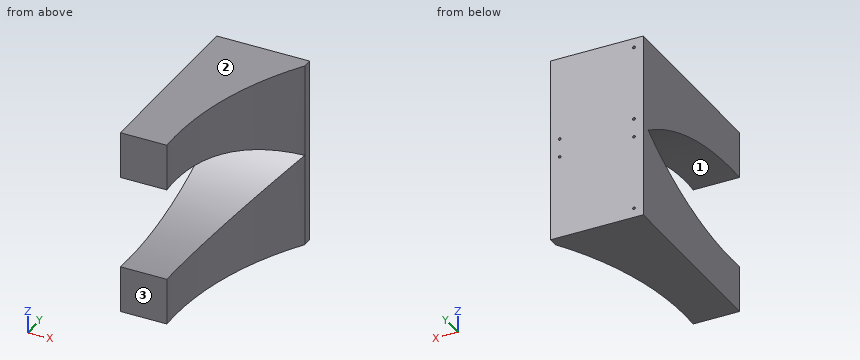
from build123d import *

# Parameters (mm, degrees)
SKETCH1_W           = 100
SKETCH1_H           = 100
BOSS_EXTRUDE1_DEPTH = 200
CUT_EXTRUDE1_DEPTH  = 200
CUT_EXTRUDE2_DEPTH  = 200
SKETCH4_R           = 1.45
CUT_EXTRUDE3_DEPTH  = 10


with BuildPart() as part:
    # Sketch1 → Boss-Extrude1 (new body)
    with BuildSketch(Plane(origin=(0, 0, 0), x_dir=(1, 0, 0), z_dir=(0, 1, 0))):
        with Locations((50, 50)):
            Rectangle(SKETCH1_W, SKETCH1_H)
    extrude(amount=-BOSS_EXTRUDE1_DEPTH)

    # Sketch2 → Cut-Extrude1 (cut)
    with BuildSketch(Plane.XY):
        with BuildLine():
            ThreePointArc((100, -10), (60.05758303, -101.067785008), (50, -200))
            Line((50, -200), (100, -200))
            Line((100, -200), (100, -10))
        make_face()
    extrude(amount=-CUT_EXTRUDE1_DEPTH, mode=Mode.SUBTRACT)

    # Sketch3 → Cut-Extrude2 (cut)
    with BuildSketch(Plane.ZY):
        with BuildLine():
            ThreePointArc((-50, -200), (-60.05758303, -101.067785008), (-100, -10))
            Line((-100, -10), (-100, -200))
            Line((-100, -200), (-50, -200))
        make_face()
    extrude(amount=-CUT_EXTRUDE2_DEPTH, mode=Mode.SUBTRACT)

    # Sketch4 → Cut-Extrude3 (cut)
    with BuildSketch(Plane(origin=(0, 0, 0), x_dir=(1, 0, 0), z_dir=(0, 1, 0))):
        with Locations((10, 90)):
            Circle(SKETCH4_R)
        with Locations((90, 90)):
            Circle(SKETCH4_R)
        with Locations((10, 10)):
            Circle(SKETCH4_R)
    extrude(amount=-CUT_EXTRUDE3_DEPTH, mode=Mode.SUBTRACT)

    # Mirror1: part across plane


with BuildPart() as part_1:
    add(part.part)
    add(part.part.mirror(Plane(origin=(0, -200, -100), x_dir=(1, 0, 0), z_dir=(0, 0, -1))))


solid = part_1.part
Input: part model. Units: mm. Frame: model coordinates. Face numbers are marked on the shaded views. Give positions to 0.01 mm unless a question says otherwise; leave off trailing zeros. Order: outer loops, then holes, each group sorted by start corner. A loop starts at its lowest first (then second) coordinate and runs counter-clockwise, first axis right, second up. Notation, with made-up numbers: (27.5, 42.5) - (81.5, 42.5) arc R16 ccw to (81.5, 51.5) - close; hole circle Ø6 at (-37.5, 48). An arc over 180 degrees is marked (long way). Answer as a JSON object with one key per item and string values. Group by question number.
Q1. Cut plane A-A, the plane y = -72. Output: boundary loops of the cut face in (x, z).
Q2. Cut plane C-C, the plane z = -17. Output: boundary loops of the cut face in (x, y), then the cut area to 3 significant figures.
Q3. Line query: probe 1 along Z at (x, y) = (10, -2.25); probe 2 along X at (y, z) = (-5, -90); probe 3 along Z at (x, y) = (90, -2). Output: solid intervals per line, ascending.
Q4. Mould query, pull axis Z, two halves, no side actions, for the marked faces 1, 2 and 3. Classes: pulls with the +Z half, pulls with the -Z half, needs draft (parallel to the pull), parting line crosses it, or undercut.
Q5. Cut plane B-B, the plane x = 20.5. Output: boundary loops of the cut face in (y, z).
Q6. Cut plane D-D, the plane y = -49.5. Output: boundary loops of the cut face in (x, z), then the cut area to 3 significant figures.
Q7. First-contact query: pin 1 Ø10 at (y, z) = (-48, -51.5) entering from +X; pin 2 Ø1.4 at (x, z) = (10.5, -110) entering from +Y; pin 3 Ø4.5 at (x, z) = (10, -110) entering from -Y. Flat tips, straight axial feed; report the tip coordinate or a pass-through.
Results:
{
 "1": {"outline": "(0, -200) - (69.21, -200) - (69.21, -130.79) - (0, -130.79) - close; (0, -69.21) - (69.21, -69.21) - (69.21, 0) - (0, 0) - close"},
 "2": {"outline": "(0, -200) - (50, -200) arc R320 cw to (100, -10) - (100, 0) - (0, 0) - close", "area": "13,200 mm^2"},
 "3": {"probe 1": "-200 to -191.45, -188.55 to -111.45, -108.55 to -91.45, -88.55 to -11.45, -8.55 to 0", "probe 2": "0 to 8.55, 11.45 to 88.55, 91.45 to 100", "probe 3": "-200 to -111.45, -108.55 to -91.45, -88.55 to 0"},
 "4": {"face 1": "undercut", "face 2": "pulls with the +Z half", "face 3": "needs draft"},
 "5": {"outline": "(-200, -200) - (0, -200) - (0, 0) - (-200, 0) - (-200, -50) arc R320 cw to (-10, -100) arc R320 cw to (-200, -150) - close"},
 "6": {"outline": "(0, -200) - (78.47, -200) - (78.47, -121.53) - (0, -121.53) - close; (0, -78.47) - (78.47, -78.47) - (78.47, 0) - (0, 0) - close", "area": "12,300 mm^2"},
 "7": {"pin 1": "x = 81.53", "pin 2": "y = -10", "pin 3": "y = -30.83"}
}
